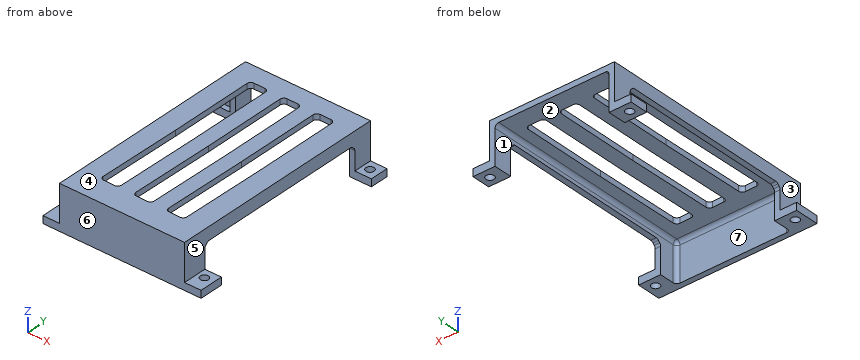
from build123d import *

# Parameters (mm, degrees)
SKETCH1_W             = 6
SKETCH1_H             = 5
SKETCH1_R             = 1.1
BOSS_EXTRUDE1_DEPTH   = 2
BOSS_EXTRUDE1_2_DEPTH = 2
BOSS_EXTRUDE1_3_DEPTH = 2
BOSS_EXTRUDE1_4_DEPTH = 2
SKETCH2_W             = 1.5
SKETCH2_H             = 5
BOSS_EXTRUDE2_DEPTH   = 10
SKETCH3_W             = 34
SKETCH3_H             = 58
BOSS_EXTRUDE3_DEPTH   = 1.5
BOSS_EXTRUDE4_DEPTH   = 1.5
CHAMFER1_SIZE         = 3
SKETCH5_W             = 1.5
SKETCH5_H             = 50
BOSS_EXTRUDE5_DEPTH   = 2
FILLET1_R             = 1
CUT_EXTRUDE1_DEPTH    = 2
FILLET2_R             = 1


with BuildPart() as part:
    # Sketch1 → Boss-Extrude1 (new body)
    with BuildSketch(Plane.XY):
        with Locations((18.5, 50.5)):
            Rectangle(SKETCH1_W, SKETCH1_H)
        with Locations((19, 50.5)):
            Circle(SKETCH1_R, mode=Mode.SUBTRACT)
    extrude(amount=BOSS_EXTRUDE1_DEPTH)



with BuildPart() as body_2:
    # Sketch1 → Boss-Extrude1 2 (new body)
    with BuildSketch(Plane.XY):
        with Locations((-18.5, 50.5)):
            Rectangle(SKETCH1_W, SKETCH1_H)
        with Locations((-19, 50.5)):
            Circle(SKETCH1_R, mode=Mode.SUBTRACT)
    extrude(amount=BOSS_EXTRUDE1_2_DEPTH)


with BuildPart() as body_3:
    # Sketch1 → Boss-Extrude1 3 (new body)
    with BuildSketch(Plane.XY):
        with Locations((18.5, -2.5)):
            Rectangle(SKETCH1_W, SKETCH1_H)
        with Locations((19, -2.5)):
            Circle(SKETCH1_R, mode=Mode.SUBTRACT)
    extrude(amount=BOSS_EXTRUDE1_3_DEPTH)


with BuildPart() as body_4:
    # Sketch1 → Boss-Extrude1 4 (new body)
    with BuildSketch(Plane.XY):
        with Locations((-18.5, -2.5)):
            Rectangle(SKETCH1_W, SKETCH1_H)
        with Locations((-19, -2.5)):
            Circle(SKETCH1_R, mode=Mode.SUBTRACT)
    extrude(amount=BOSS_EXTRUDE1_4_DEPTH)


with BuildPart() as part_1:
    add(part.part)

    add(body_2.part)  # Boss-Extrude2 merges body 2

    add(body_3.part)  # Boss-Extrude2 merges body 3

    add(body_4.part)  # Boss-Extrude2 merges body 4
    # Sketch2 → Boss-Extrude2 (add)
    with BuildSketch(Plane.XY.offset(2)):
        with Locations((16.25, 50.5)):
            Rectangle(SKETCH2_W, SKETCH2_H)
        with Locations((16.25, -2.5)):
            Rectangle(SKETCH2_W, SKETCH2_H)
        with Locations((-16.25, -2.5)):
            Rectangle(SKETCH2_W, SKETCH2_H)
        with Locations((-16.25, 50.5)):
            Rectangle(SKETCH2_W, SKETCH2_H)
    extrude(amount=BOSS_EXTRUDE2_DEPTH)

    # Sketch3 → Boss-Extrude3 (add)
    with BuildSketch(Plane.XY.offset(12)):
        with Locations((0, 24)):
            Rectangle(SKETCH3_W, SKETCH3_H)
    extrude(amount=-BOSS_EXTRUDE3_DEPTH)

    # Sketch4 → Boss-Extrude4 (add)
    with BuildSketch(Plane.XZ.offset(5)):
        Polygon((-15.5, 0), (15.5, 0), (21.5, 0), (21.5, 2), (17, 2), (17, 12), (-17, 12), (-17, 2), (-21.5, 2), (-21.5, 0), align=None)
    extrude(amount=BOSS_EXTRUDE4_DEPTH)

    # Chamfer1
    chamfer1_edges = [part_1.edges().sort_by_distance(p)[0] for p in [
        (16.25, 48, 10.5),
        (-16.25, 48, 10.5),
        (16.25, 0, 10.5),
        (-16.25, 0, 10.5),
    ]]
    chamfer(chamfer1_edges, length=CHAMFER1_SIZE)

    # Sketch5 → Boss-Extrude5 (add)
    with BuildSketch(Plane(origin=(0, 0, 10.5), x_dir=(-1, 0, 0), z_dir=(0, 0, -1))):
        with Locations((16.25, 24)):
            Rectangle(SKETCH5_W, SKETCH5_H)
        with Locations((-16.25, 24)):
            Rectangle(SKETCH5_W, SKETCH5_H)
    extrude(amount=BOSS_EXTRUDE5_DEPTH)

    # Fillet1
    fillet1_edges = [part_1.edges().sort_by_distance(p)[0] for p in [
        (-16.25, 0, 7.5),
        (-16.25, 48, 7.5),
        (16.25, 0, 7.5),
        (16.25, 48, 7.5),
        (16.25, 47, 8.5),
        (16.25, 1, 8.5),
        (-16.25, 1, 8.5),
        (15.5, 24, 10.5),
        (-15.5, 24, 10.5),
        (15.5, -5, 5.25),
        (0, -5, 10.5),
        (-15.5, -5, 5.25),
    ]]
    fillet(fillet1_edges, radius=FILLET1_R)

    # Sketch6 → Cut-Extrude1 (cut)
    with BuildSketch(Plane(origin=(0, 0, 10.5), x_dir=(-1, 0, 0), z_dir=(0, 0, -1))):
        Polygon((-6.5, 48.033502568), (-11.5, 48.033502568), (-11.5, 24.033502568), (-11.207624805, 0.035283535), (-6.207995839, 0.096195034), (-6.5, 24.063959447), align=None)
        Polygon((-2.5, 48.033502568), (-2.5, 24.088324951), (-2.208292667, 0.144924233), (2.791336298, 0.205835732), (2.5, 24.11878183), (2.5, 48.033502568), align=None)
        Polygon((11.5, 48.033502568), (6.5, 48.033502568), (6.5, 24.143147334), (6.79103947, 0.254564931), (11.790668435, 0.31547643), (11.5, 24.173604214), align=None)
    extrude(amount=-CUT_EXTRUDE1_DEPTH, mode=Mode.SUBTRACT)

    # Fillet2
    fillet2_edges = [part_1.edges().sort_by_distance(p)[0] for p in [
        (11.207624805, 0.035283535, 11.25),
        (11.5, 48.033502568, 11.25),
        (6.5, 48.033502568, 11.25),
        (6.207995839, 0.096195034, 11.25),
        (-2.791336298, 0.205835732, 11.25),
        (2.208292667, 0.144924233, 11.25),
        (2.5, 48.033502568, 11.25),
        (-2.5, 48.033502568, 11.25),
        (-6.79103947, 0.254564931, 11.25),
        (-6.5, 48.033502568, 11.25),
        (-11.5, 48.033502568, 11.25),
        (-11.790668435, 0.31547643, 11.25),
    ]]
    fillet(fillet2_edges, radius=FILLET2_R)


solid = part_1.part
Part model, mm, in its own coordinate system. Face numbers are marked on the shaded views. A direction names the side the tool comes from. Coordinates: 2 decimals unless noted, no trailing zeros. Order: outer loops, then holes, each group sorted by start corner. A loop starts at its lowest first (then second) coordinate and runs counter-clockwise, first axis right, second up.
(1) Pull direction X, two halves, no side cores. Call the marked faces 1, 2, 3 and 4: pulls with the +X half, pulls with the -X half, needs draft (parallel to the pull), parting line crosses it, or undercut.
Check sheet entries:
face 1: undercut
face 2: undercut
face 3: pulls with the -X half
face 4: needs draft
(2) Tool access for the marked faces 5, 6 and 7: list every direction of +Z, -Z, +X, -X, +Y, -Y with a clear straight run to the whole face (end or side of a thin tool).
Check sheet entries:
face 5: +Z, +X, +Y, -Y
face 6: +Z, -Z, +X, -X, -Y
face 7: -Z, +Y
(3) Probe L1, parallel to Y at x = -19, z = 1.4; L2, parallel to X at y = 30, z = 9; L3, parallel to Y at x = 16.5, z = 5.75. List the from-to ranges inside material, lowest first.
Check sheet entries:
L1: y = -6.5 to -3.6, -1.4 to 0, 48 to 49.4, 51.6 to 53
L2: x = -17 to -15.5, 15.5 to 17
L3: y = -6.5 to 0, 48 to 53
(4) Slice it at A-A, the plane y = 43. Write the cut outline in (x, z).
Check sheet entries:
outline: (-17, 8.5) - (-15.5, 8.5) - (-15.5, 9.5) arc R1 cw to (-14.5, 10.5) - (-11.5, 10.5) - (-11.5, 12) - (-17, 12) - close; (-6.5, 10.5) - (-2.5, 10.5) - (-2.5, 12) - (-6.5, 12) - close; (2.5, 10.5) - (6.5, 10.5) - (6.5, 12) - (2.5, 12) - close; (11.5, 10.5) - (14.5, 10.5) arc R1 cw to (15.5, 9.5) - (15.5, 8.5) - (17, 8.5) - (17, 12) - (11.5, 12) - close
(5) Slice it at B-B, the plane z = 4.25. Write the cut outline in (x, y).
Check sheet entries:
outline: (-17, -6.5) - (17, -6.5) - (17, 0) - (15.5, 0) - (15.5, -4) arc R1 cw to (14.5, -5) - (-14.5, -5) arc R1 cw to (-15.5, -4) - (-15.5, 0) - (-17, 0) - close; (-17, 48) - (-15.5, 48) - (-15.5, 53) - (-17, 53) - close; (15.5, 48) - (17, 48) - (17, 53) - (15.5, 53) - close
(6) Pin check, flat tips, straight feed: pin 1 Ø0.8 at (y, z) = (40, 11.5) entering from -X; pin 2 Ø3 at (x, y) = (19, -2.5) entering from +Z; pin 3 Ø3 at (x, z) = (6.5, 3) entering from +Y; pin 4 Ø5 at (x, z) = (13.5, 8) entering from +Y. Stop position of each tip, or through.
Check sheet entries:
pin 1: stops at x = -17
pin 2: stops at z = 2
pin 3: stops at y = -5
pin 4: stops at y = 53
(7) Slice it at D-D, the plane y = -2.5. Write the cut outline in (x, z).
Check sheet entries:
outline: (-21.5, 0) - (-20.1, 0) - (-20.1, 2) - (-21.5, 2) - close; (-17.9, 0) - (-15.5, 0) - (-15.5, 9.5) arc R1 cw to (-14.5, 10.5) - (14.5, 10.5) arc R1 cw to (15.5, 9.5) - (15.5, 0) - (17.9, 0) - (17.9, 2) - (17, 2) - (17, 12) - (-17, 12) - (-17, 2) - (-17.9, 2) - close; (20.1, 0) - (21.5, 0) - (21.5, 2) - (20.1, 2) - close
(8) Slice it at C-C, the plane x = 19. Write the cut outline in (y, z), and give its area (3 significant figures).
Check sheet entries:
outline: (-6.5, 0) - (-3.6, 0) - (-3.6, 2) - (-6.5, 2) - close; (-1.4, 0) - (0, 0) - (0, 2) - (-1.4, 2) - close; (48, 0) - (49.4, 0) - (49.4, 2) - (48, 2) - close; (51.6, 0) - (53, 0) - (53, 2) - (51.6, 2) - close
area: 14.2 mm2
